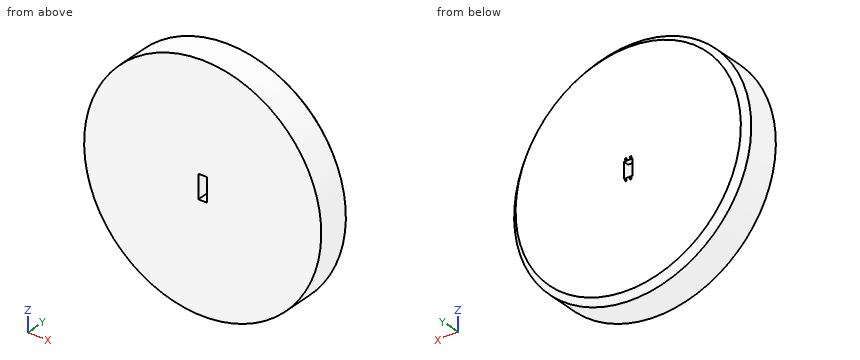
```python
from build123d import *

# Parameters (mm, degrees)
SKETCH1_R           = 200
BOSS_EXTRUDE1_DEPTH = 65
SKETCH2_W           = 15
SKETCH2_H           = 27
CUT_EXTRUDE1_DEPTH  = 291.215437219
SKETCH3_W           = 15
SKETCH3_H           = 40
CUT_EXTRUDE2_DEPTH  = 55
CHAMFER1_SIZE       = 10
SKETCH4_R           = 1.5
CUT_EXTRUDE3_DEPTH  = 289.140590684


with BuildPart() as part:
    # Sketch1 → Boss-Extrude1 (new body)
    with BuildSketch(Plane(origin=(0, 0, 0), x_dir=(1, 0, 0), z_dir=(0, 1, 0))):
        with Locations(Location((0, 0, 0), (0, 0, 270))):
            Circle(SKETCH1_R)
    extrude(amount=BOSS_EXTRUDE1_DEPTH)

    # Sketch2 → Cut-Extrude1 (cut, through all)
    with BuildSketch(Plane(origin=(0, 65, 0), x_dir=(1, 0, 0), z_dir=(0, 1, 0))):
        Rectangle(SKETCH2_W, SKETCH2_H)
    extrude(amount=-CUT_EXTRUDE1_DEPTH, mode=Mode.SUBTRACT)

    # Sketch3 → Cut-Extrude2 (cut)
    with BuildSketch(Plane.XZ):
        Rectangle(SKETCH3_W, SKETCH3_H)
    extrude(amount=-CUT_EXTRUDE2_DEPTH, mode=Mode.SUBTRACT)

    # Chamfer1
    chamfer1_edges = [part.edges().sort_by_distance(p)[0] for p in [
        (0, 65, -200),
    ]]
    chamfer(chamfer1_edges, length=CHAMFER1_SIZE)

    # Sketch4 → Cut-Extrude3 (cut, through all)
    with BuildSketch(Plane(origin=(0, 55, 0), x_dir=(-1, 0, 0), z_dir=(0, -1, 0))):
        with Locations(Location((4, -16.75, 0), (0, 0, 90))):
            Circle(SKETCH4_R)
        with Locations(Location((-4, -16.75, 0), (0, 0, 270))):
            Circle(SKETCH4_R)
        with Locations(Location((4, 16.75, 0), (0, 0, 270))):
            Circle(SKETCH4_R)
        with Locations(Location((-4, 16.75, 0), (0, 0, 90))):
            Circle(SKETCH4_R)
    extrude(amount=-CUT_EXTRUDE3_DEPTH, mode=Mode.SUBTRACT)


solid = part.part
```
The model under review builds one solid part; all positions refer to its coordinate system, in mm. Round coordinates to 2 decimals unless told otherwise and drop trailing zeros. Order: outer loops, then holes, each group sorted by start corner. A loop starts at its lowest first (then second) coordinate and runs counter-clockwise, first axis right, second up. Notation, with made-up numbers: (-32.5, 59) - (4.5, 59) arc R22 cw to (4.5, 71) - close; hole circle Ø10 at (24, -26). An arc over 180 degrees is marked (long way). Answer in a Markdown table with one row per item.
(1) Clearance check with flat-ended pins moving along their axes: P1, Ø4, axis at x = 4, z = -16.75, coming from the +Y side; P2, Ø5, axis at x = 2.5, y = 61, coming from the +Z side; P3, Ø1.5, axis at y = 56, z = -9.5, coming from the -X side; P4, Ø8, axis at x = 1, y = 62, coming from the -Z side. State where each tip first meets the part, or that it passes through.
Result set:
| item | result |
|---|---|
| P1 | stops at y = 65 |
| P2 | stops at z = 196.48 |
| P3 | stops at x = -199.52 |
| P4 | stops at z = -197 |
(2) For line 1 (X direction, y = 60.25, z = 16.75); line 2 (X direction, y = 7.5, z = 3.5); line 3 (X direction, y = 57, z = -16.75), list the stretches that pass through material, from the lowest coordinate up. Write a range as from..to.
Result set:
| item | result |
|---|---|
| line 1 | x = -194.03..-5.5, -2.5..2.5, 5.5..194.03 |
| line 2 | x = -199.97..-7.5, 7.5..199.97 |
| line 3 | x = -197.29..-5.5, -2.5..2.5, 5.5..197.29 |
(3) Take a section at A-A on y = 22. Write out the cut boundary in (x, z).
Result set:
| item | result |
|---|---|
| outline | circle Ø400 at (0, 0); hole (-7.5, -20) - (7.5, -20) - (7.5, 20) - (-7.5, 20) - close |
